```python
from build123d import *

# Parameters (mm, degrees)
BOX081_W                          = 90
BOX081_H                          = 9
BOX081_DEPTH                      = 4
BOX080_W                          = 10
BOX080_H                          = 3
BOX080_DEPTH                      = 4
BOX079_W                          = 40
BOX079_H                          = 10
BOX079_DEPTH                      = 10
CYLINDER143_R                     = 3.25
CYLINDER143_DEPTH                 = 3.5
CYLINDER144_R                     = 0.6
CYLINDER144_DEPTH                 = 9.5
CYLINDER142_R                     = 0.6
CYLINDER142_DEPTH                 = 9.5
CYLINDER141_R                     = 3.25
CYLINDER141_DEPTH                 = 3.5
PAD014_DEPTH                      = 4
FILLET078_R                       = 3
PART_MIRRORING003_PLACEMENT_ANGLE = 180
BOX078_W                          = 40
BOX078_H                          = 10
BOX078_DEPTH                      = 10
CYLINDER137_R                     = 3.25
CYLINDER137_DEPTH                 = 3.5
CYLINDER140_R                     = 0.6
CYLINDER140_DEPTH                 = 9.5
CYLINDER138_R                     = 0.6
CYLINDER138_DEPTH                 = 9.5
CYLINDER139_R                     = 3.25
CYLINDER139_DEPTH                 = 3.5
PAD013_DEPTH                      = 4
FILLET077_R                       = 3


with BuildPart() as obj1:
    # Box081 → Box081 (new body)
    with BuildSketch(Plane(origin=(-63, -38.5, -41), x_dir=(1, 0, 0), z_dir=(0, 0, 1))):
        with Locations((45, 4.5)):
            Rectangle(BOX081_W, BOX081_H)
    extrude(amount=BOX081_DEPTH)


with BuildPart() as obj2:
    # Box080 → Box080 (new body)
    with BuildSketch(Plane(origin=(-23, -35.5, -38), x_dir=(1, 0, 0), z_dir=(0, 0, 1))):
        with Locations((5, 1.5)):
            Rectangle(BOX080_W, BOX080_H)
    extrude(amount=BOX080_DEPTH)


with BuildPart() as obj3:
    # Box079 → Box079 (new body)
    with BuildSketch(Plane(origin=(-14, -72, -42), x_dir=(1, 0, 0), z_dir=(0, 0, 1))):
        with Locations((20, 5)):
            Rectangle(BOX079_W, BOX079_H)
    extrude(amount=BOX079_DEPTH)


with BuildPart() as zylinder143:
    # Cylinder143 → Cylinder143 (new body)
    with BuildSketch(Plane(origin=(-52.5, 23, -36), x_dir=(1, 0, 0), z_dir=(0, 0, 1))):
        Circle(CYLINDER143_R)
    extrude(amount=CYLINDER143_DEPTH)


with BuildPart() as zylinder144:
    # Cylinder144 → Cylinder144 (new body)
    with BuildSketch(Plane(origin=(16.5, 23, -39), x_dir=(1, 0, 0), z_dir=(0, 0, 1))):
        Circle(CYLINDER144_R)
    extrude(amount=CYLINDER144_DEPTH)


with BuildPart() as zylinder142:
    # Cylinder142 → Cylinder142 (new body)
    with BuildSketch(Plane(origin=(-52.5, 23, -39), x_dir=(1, 0, 0), z_dir=(0, 0, 1))):
        Circle(CYLINDER142_R)
    extrude(amount=CYLINDER142_DEPTH)


with BuildPart() as fusion089:
    # Cylinder141 → Cylinder141 (new body)
    with BuildSketch(Plane(origin=(16.5, 23, -36), x_dir=(1, 0, 0), z_dir=(0, 0, 1))):
        Circle(CYLINDER141_R)
    extrude(amount=CYLINDER141_DEPTH)

    # Fusion089: union Zylinder143, Zylinder144, Zylinder142
    add(zylinder143.part)
    add(zylinder144.part)
    add(zylinder142.part)


with BuildPart() as cut068:
    # Sketch014 → Pad014 (new body)
    with BuildSketch(Plane.XY):
        with BuildLine():
            add(Edge.make_bspline(
                [(-48.5, 19), (-18, 24), (12.5, 19)],
                knots=[0, 0, 0, 1, 1, 1], degree=2))
            Line((-48.5, 19), (-57, 19))
            Line((-57, 19), (-57, 27))
            Line((-57, 27), (-48.5, 27))
            add(Edge.make_bspline(
                [(-48.5, 27), (-18, 22), (12.5, 27)],
                knots=[0, 0, 0, 1, 1, 1], degree=2))
            Line((12.5, 27), (21, 27))
            Line((21, 27), (21, 19))
            Line((21, 19), (12.5, 19))
        make_face()
    extrude(amount=PAD014_DEPTH)


with BuildPart() as cut068_1:
    # Body005 placement: moved
    add(cut068.part.moved(Location((0, 0, -38))))

    # Cut069: cut Fusion089
    add(fusion089.part, mode=Mode.SUBTRACT)

    # Fillet078
    fillet078_edges = [cut068_1.edges().sort_by_distance(p)[0] for p in [
        (-57, 19, -36),
        (21, 19, -36),
        (-57, 27, -36),
        (21, 27, -36),
    ]]
    fillet(fillet078_edges, radius=FILLET078_R)


with BuildPart() as cut068_2:
    # Fillet078 placement: moved
    add(cut068_1.part.moved(Location((0, -90, 0))))

    # Cut068: cut obj3
    add(obj3.part, mode=Mode.SUBTRACT)


with BuildPart() as cut068_3:
    # Cut068 placement: moved
    add(cut068_2.part.moved(Location((-5, 35, 0))))


with BuildPart() as part_mirroring003:
    # Part__Mirroring003: instance of Cut068
    add(cut068_3.part.mirror(Plane(origin=(-40.5, -8e-06, -36), x_dir=(1, 0, 0), z_dir=(0, 1, 0))))


with BuildPart() as part_mirroring003_1:
    # Part__Mirroring003 placement: moved
    add(part_mirroring003.part.moved(Location((-36, 9, 0))).rotate(Axis((-36, 9, 0), (0, 0, 1)), PART_MIRRORING003_PLACEMENT_ANGLE))


with BuildPart() as obj4:
    # Box078 → Box078 (new body)
    with BuildSketch(Plane(origin=(-14, -72, -42), x_dir=(1, 0, 0), z_dir=(0, 0, 1))):
        with Locations((20, 5)):
            Rectangle(BOX078_W, BOX078_H)
    extrude(amount=BOX078_DEPTH)


with BuildPart() as zylinder137:
    # Cylinder137 → Cylinder137 (new body)
    with BuildSketch(Plane(origin=(-52.5, 23, -36), x_dir=(1, 0, 0), z_dir=(0, 0, 1))):
        Circle(CYLINDER137_R)
    extrude(amount=CYLINDER137_DEPTH)


with BuildPart() as zylinder140:
    # Cylinder140 → Cylinder140 (new body)
    with BuildSketch(Plane(origin=(16.5, 23, -39), x_dir=(1, 0, 0), z_dir=(0, 0, 1))):
        Circle(CYLINDER140_R)
    extrude(amount=CYLINDER140_DEPTH)


with BuildPart() as zylinder138:
    # Cylinder138 → Cylinder138 (new body)
    with BuildSketch(Plane(origin=(-52.5, 23, -39), x_dir=(1, 0, 0), z_dir=(0, 0, 1))):
        Circle(CYLINDER138_R)
    extrude(amount=CYLINDER138_DEPTH)


with BuildPart() as fusion088:
    # Cylinder139 → Cylinder139 (new body)
    with BuildSketch(Plane(origin=(16.5, 23, -36), x_dir=(1, 0, 0), z_dir=(0, 0, 1))):
        Circle(CYLINDER139_R)
    extrude(amount=CYLINDER139_DEPTH)

    # Fusion088: union Zylinder137, Zylinder140, Zylinder138
    add(zylinder137.part)
    add(zylinder140.part)
    add(zylinder138.part)


with BuildPart() as cut070:
    # Sketch013 → Pad013 (new body)
    with BuildSketch(Plane.XY):
        with BuildLine():
            add(Edge.make_bspline(
                [(-48.5, 19), (-18, 24), (12.5, 19)],
                knots=[0, 0, 0, 1, 1, 1], degree=2))
            Line((-48.5, 19), (-57, 19))
            Line((-57, 19), (-57, 27))
            Line((-57, 27), (-48.5, 27))
            add(Edge.make_bspline(
                [(-48.5, 27), (-18, 22), (12.5, 27)],
                knots=[0, 0, 0, 1, 1, 1], degree=2))
            Line((12.5, 27), (21, 27))
            Line((21, 27), (21, 19))
            Line((21, 19), (12.5, 19))
        make_face()
    extrude(amount=PAD013_DEPTH)


with BuildPart() as cut070_1:
    # Body004 placement: moved
    add(cut070.part.moved(Location((0, 0, -38))))

    # Cut066: cut Fusion088
    add(fusion088.part, mode=Mode.SUBTRACT)

    # Fillet077
    fillet077_edges = [cut070_1.edges().sort_by_distance(p)[0] for p in [
        (-57, 19, -36),
        (21, 19, -36),
        (-57, 27, -36),
        (21, 27, -36),
    ]]
    fillet(fillet077_edges, radius=FILLET077_R)


with BuildPart() as cut070_2:
    # Fillet077 placement: moved
    add(cut070_1.part.moved(Location((0, -90, 0))))

    # Cut067: cut obj4
    add(obj4.part, mode=Mode.SUBTRACT)


with BuildPart() as cut070_3:
    # Cut067 placement: moved
    add(cut070_2.part.moved(Location((-5, 44, 0))))

    # Fusion090: union Part__Mirroring003
    add(part_mirroring003_1.part)


with BuildPart() as cut070_4:
    # Fusion090 placement: moved
    add(cut070_3.part.moved(Location((0, -11, 0))))

    # Fusion091: union obj2
    add(obj2.part)

    # Cut070: cut obj1
    add(obj1.part, mode=Mode.SUBTRACT)


solid = cut070_4.part
```
Source: CAD feature listing. Evaluate the final solid. Frame: model axes, mm. A direction names the side the tool comes from. Give positions to 0.01 mm unless a question says otherwise; leave off trailing zeros.
(1) Pull-direction query (Y, two-part tool) for faces 5 (the face through (-19, -34, -37)), 6 (the face through (22.205, -37.173, -35.014)), 7 (the face through (20, -30, -36)); classes: +Y half, -Y half, draft (parallel to the pull), parting line (faces both ways), or undercut.
(2) Access query for faces 1 (the face through (-18, -32.5, -36)), 2 (the face through (26, -34, -36)), 3 (the face through (22, -35, -36)), 4 (the face through (-18, -35.5, -36)). Directions: +Z, -Z, +X, -X, +Y, -Y. A direction counts if a zero-diameter tool reaches every point of the face in a straight line with its end or side. Return the directions, or none.
(3) Contact query for flat-ended pins moving along their axis: P1, Ø1, axis at x = -26, z = -36.5, coming from the +Y side; P2, Ø1.4, axis at x = 21.5, y = -34, coming from the +Z side; P3, Ø1.5, axis at y = -36, z = -36.5, coming from the +X side. Output: stop coordinate, or through.
(4) Section query A-A (z = -34.85). State how many separate pieces and enclosed holes the cut face has, plus the area to 3 significant figures.
(5) Material intervals for line 1 along X through (y, z) = (-34, -36.7); line 2 along X through (y, z) = (-33, -35.9); line 3 along Y through (x, z) = (21.5, -35.35), sorted ascending.
Outcome:
1. face 5: draft
1. face 6: undercut
1. face 7: +Y half
2. face 1: +Z, -Z, +Y
2. face 2: +Z, -Z, +X, +Y, -Y
2. face 3: +Z
2. face 4: +Z, -Z, -Y
3. P1: stops at y = -32.47
3. P2: stops at z = -36
3. P3: stops at x = 25.99
4. separate pieces: 1
4. enclosed holes: 2
4. area: 377 mm2
5. line 1: x = -62 to -58.1, -56.9 to 20.9, 22.1 to 26
5. line 2: x = -62 to -60.59, -54.41 to 18.41, 24.59 to 26
5. line 3: y = -38 to -37.25, -30.75 to -30
